Autodesk Inventor part; units mm, degrees
ref_plane "YZ Plane" through (0, 0, 0) normal (1, 0, 0) x (0, 1, 0)
ref_plane "XZ Plane" through (0, 0, 0) normal (0, 1, 0) x (-1, 0, 0)
ref_plane "XY Plane" through (0, 0, 0) normal (0, 0, 1) x (1, 0, 0)
sketch "Sketch5" plane through (0, 0, 0) normal (0, 0, 1) x (1, 0, 0)
  line L0 (0, 0) -> (-60, 0)
  line L1 (-60, 0) -> (-60, 60)
  line L2 (-60, 60) -> (0, 60)
  line L3 (0, 60) -> (0, 0)
  dimension "d55" = 60
  dimension "d56" = 60
extrude "Extrusion4" add sketch "Sketch5" along normal blind 35.4
sketch "Sketch6" plane through (0, 0, 0) normal (1, 0, 0) x (0, 0, -1)
  line L0 (-35.4, 60) -> (-35.4, 0)
  line L1 (-35.4, 60) -> (-25.4, 60)
  line L2 (-25.4, 60) -> (-25.4, 50)
  line L3 (-25.4, 50) -> (-35.4, 50)
  line L4 (-35.4, 50) -> (-35.4, 60)
  line L5 (-25.4, 50) -> (-9.4, 50)
  line L6 (-9.4, 50) -> (-9.4, 29.6)
  line L7 (-9.4, 29.6) -> (-25.4, 29.6)
  line L8 (-25.4, 29.6) -> (-25.4, 50)
  point P0 (0, 0)
  dimension "d61" = 10
  dimension "d62" = 10
  dimension "d65" = 16
  dimension "d66" = 20.4
extrude "Extrusion5" cut sketch "Sketch6" against normal blind 50 contours L5 L6 L7 L8
sketch "Sketch7" plane through (-60, 0, 0) normal (-1, 0, 0) x (0, 0, 1)
  line L0 (0, 0) -> (0, 60)
  line L1 (0, 60) -> (10, 60)
  line L2 (10, 60) -> (10, 50)
  line L3 (10, 50) -> (0, 50)
  line L4 (0, 50) -> (0, 60)
  line L5 (10, 50) -> (25, 50)
  line L6 (25, 50) -> (25, 30)
  line L7 (25, 30) -> (10, 30)
  line L8 (10, 30) -> (10, 50)
  dimension "d68" = 10
  dimension "d69" = 10
  dimension "d70" = 15
  dimension "d71" = 20
extrude "Extrusion6" add sketch "Sketch7" along normal blind 50 contours L5 L6 L7 L8
fillet "Fillet5" radius 2 5 edges at (-85, 50, 25) (-85, 30, 25) (-30, 60, 35.4) (-25, 29.6, 25.4) (-25, 50, 25.4)
properties part number "Clasp"
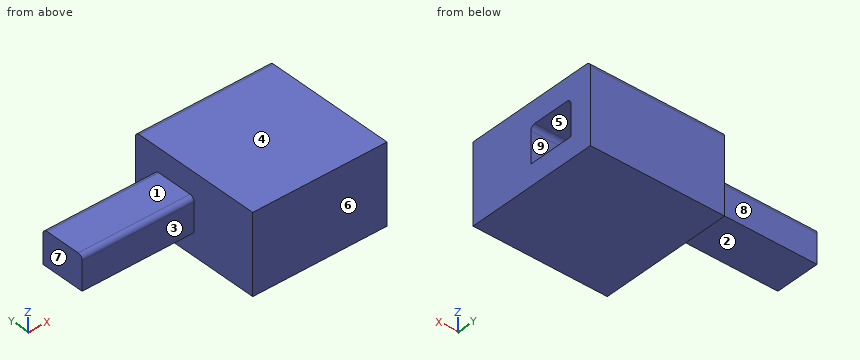
Work out the finished part from the listing and answer in its coordinate system (mm). Face numbers are marked on the shaded views. A direction names the side the tool comes from. Round coordinates to 2 decimals unless told otherwise and drop trailing zeros. Loops run counter-clockwise (first coordinate to the right, second up) from the corner with the lowest first, then second, coordinate; pieces in that order, holes last. Notation, with made-up numbers: (-7.5, 28.25) -> (12.5, 28.25) arc R18 ccw to (12.5, 37.25) -> close; hole circle Ø2 at (28, -11). An arc over 180 degrees is marked (long way). Use one line per item in the form item = value.
(1) Find section B-B on x = -27. Give the vertices of the cut face in (y, z), then the cut area to 3 significant figures.
Answer list:
outline = (0, 0) -> (60, 0) -> (60, 33.4) arc R2 ccw to (58, 35.4) -> (0, 35.4) -> close; hole (29.6, 9.4) -> (50, 9.4) -> (50, 23.4) arc R2 ccw to (48, 25.4) -> (31.6, 25.4) arc R2 ccw to (29.6, 23.4) -> close
area = 1,800 mm2
(2) For a pull along Y with two mould halves and no side action, classify the marked faces 6, 7, 8 and 9 as released by +Y, released by -Y, zero draft, split by the parting line, or undercut.
Answer list:
face_6 = released by -Y
face_7 = zero draft
face_8 = released by +Y
face_9 = undercut
(3) Flat-ended cylindrical pins translate along their axes: P1, Ø3, axis at y = 33, z = 13, coming from the +X side; P2, Ø10.5, axis at x = -92.5, z = 19.5, coming from the +Y side; P3, Ø16, axis at x = -74, y = 42.5, coming from the -Z side. Find the tip coordinate at first contact, or state that the pin passes through.
Answer list:
P1 = -50
P2 = 50
P3 = 10
(4) Find section A-A on y = 36. Give the vertices of the cut face in (x, z), then the cut area to 3 significant figures.
Answer list:
outline = (-110, 10) -> (-60, 10) -> (-60, 0) -> (0, 0) -> (0, 9.4) -> (-50, 9.4) -> (-50, 25.4) -> (0, 25.4) -> (0, 35.4) -> (-60, 35.4) -> (-60, 25) -> (-110, 25) -> close
area = 2,070 mm2
(5) Find section D-D on x = -65. Give the vertices of the cut face in (y, z).
Answer list:
outline = (30, 10) -> (50, 10) -> (50, 23) arc R2 ccw to (48, 25) -> (32, 25) arc R2 ccw to (30, 23) -> close
(6) A tool of negligible diameter and unlimited length cuts with its end or side. For the marked faces 1, 2, 3, 4 and 5, from which of +Z, -Z, +X, -X, +Y, -Y can it reach the whole face along a straight path? Write none if from no direction.
Answer list:
face_1 = +Z, -X, +Y, -Y
face_2 = -Z, -X, +Y, -Y
face_3 = +Z, -Z, -X, -Y
face_4 = +Z, +X, -X, +Y, -Y
face_5 = +X
(7) Straight lines are drawn through the part: line 1 (X direction, y = 57.5, z = 3.5); line 2 (Y direction, x = -6, z = 12); line 3 (Y direction, x = -87, z = 12.5). For each, find the intervals that lie inside material, in ascending order.
Answer list:
line_1 = -60 to 0
line_2 = 0 to 29.6, 50 to 60
line_3 = 30 to 50
(8) Find section C-C on z = 17.5. Give the vertices of the cut face in (x, y), then the cut area to 3 significant figures.
Answer list:
outline = (-110, 30) -> (-60, 30) -> (-60, 0) -> (0, 0) -> (0, 29.6) -> (-50, 29.6) -> (-50, 50) -> (0, 50) -> (0, 60) -> (-60, 60) -> (-60, 50) -> (-110, 50) -> close
area = 3,580 mm2
